For this review, use the dimensioned drawing (mm, ordinates from the lowest corner) and the shaded views. A direction names the side the tool comes from. Round coordinates to 2 decimals unless told otherwise and drop trailing zeros. Order: outer loops, then holes, each group sorted by start corner. A loop starts at its lowest first (then second) coordinate and runs counter-clockwise, first axis right, second up. Notation, with made-up numbers: M 12.25,-27.5 L 47.25,-27.5 A13 cw 47.25,-23.5 Z; hole C 12.5,2 d8. An arc over 180 degrees is marked long. Answer as CSV lines item,"result". Start each with the question number.
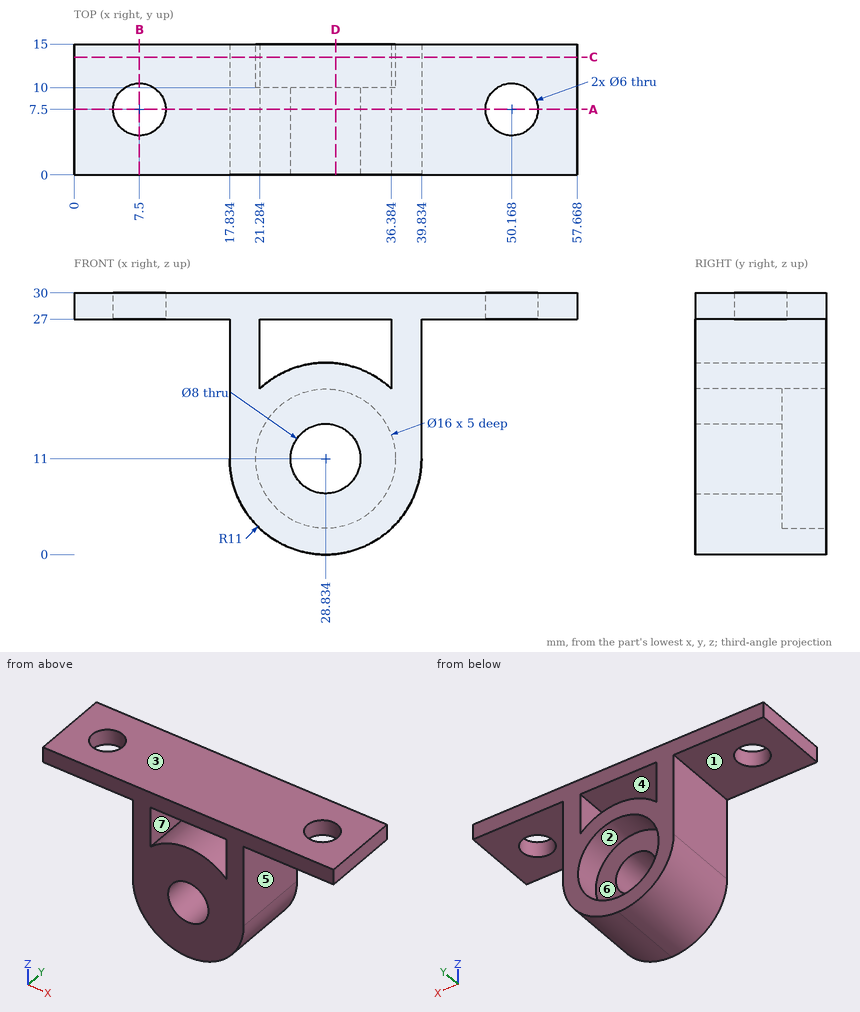
Item 1: Consider section B-B (x = 7.5). State the section outline as (y, z) points, and give its area (3 significant figures).
Item 2: For pin 1 (7.5 mm diameter, centred on x = 51, y = 8, fed in from -Z); pin 2 (5 mm diameter, centred on y = 13, z = 20.5, fed in from -X); pin 3 (2.5 mm diameter, centred on y = 7, z = 22.5, fed in from +X), all flat-tipped, find the tip position at first contact; note any pin that passes through.
Item 3: Consider section D-D (x = 30). State the section outline as (y, z) points (1 decimal).
Item 4: The part is to be moulded in two halves that separate along Z. For the marked faces 1, 2, 3 and 4, say which applies: +Z half, -Z half, draft (parallel to the pull), parting line (faces both ways), or undercut.
Item 5: Consider section A-A (y = 7.5). State the section outline as (x, z) points.
Item 6: Consider section C-C (y = 13.5). State the section outline as (x, z) points.
Item 7: Tool access review of the marked faces 5, 6 and 7: name each direction out of +Z, -Z, +X, -X, +Y, -Y from which nothing blocks a thin tool from reaching the whole face with its end or side.
Item 8: Wall thickness on probe 1 along X at (y, z) = (2.5, 19.5) (1 decimal); probe 2 along X at (y, z) = (6.5, 22.75); probe 3 along Z at (x, y) = (17, 8.25): over which ranges is each line inside the solid? List them lowest first. Write a range as [from, to].
Reported:
1,outline,"M 0,27 L 4.5,27 L 4.5,30 L 0,30 Z; M 10.5,27 L 15,27 L 15,30 L 10.5,30 Z"
1,area,"27.0 mm²"
2,pin 1,"stops at z = 27"
2,pin 2,"stops at x = 17.83"
2,pin 3,"stops at x = 39.83"
3,outline,"M 0,0.1 L 15,0.1 L 15,3.1 L 10,3.1 L 10,7.2 L 0,7.2 Z; M 0,14.8 L 10,14.8 L 10,18.9 L 15,18.9 L 15,21.9 L 0,21.9 Z; M 0,27 L 15,27 L 15,30 L 0,30 Z"
4,face 1,"-Z half"
4,face 2,"undercut"
4,face 3,"+Z half"
4,face 4,"undercut"
5,outline,"M 0,27 L 4.5,27 L 4.5,30 L 0,30 Z; M 10.5,27 L 17.83,27 L 17.83,11 A11 ccw 39.83,11 L 39.83,27 L 47.17,27 L 47.17,30 L 10.5,30 Z; M 53.17,27 L 57.67,27 L 57.67,30 L 53.17,30 Z; hole M 21.28,19 A11 cw 36.38,19 L 36.38,27 L 21.28,27 Z; hole C 28.83,11 d8"
6,outline,"M 0,27 L 17.83,27 L 17.83,11 A11 ccw 39.83,11 L 39.83,27 L 57.67,27 L 57.67,30 L 0,30 Z; hole C 28.83,11 d16; hole M 21.28,19 A11 cw 36.38,19 L 36.38,27 L 21.28,27 Z"
7,face 5,"-Z, +X, +Y, -Y"
7,face 6,"+Y"
7,face 7,"+Y, -Y"
8,probe 1,"x = [17.8, 21.3], [21.9, 35.8], [36.4, 39.8]"
8,probe 2,"x = [17.83, 21.28], [36.38, 39.83]"
8,probe 3,"z = [27, 30]"
